```python
from build123d import *

# Parameters (mm, degrees)
SKETCH_W         = 40
SKETCH_H         = 87
PAD_DEPTH        = 5
SKETCH001_R      = 1.35
POCKET_DEPTH     = 10.001
SKETCH009_R      = 1.6
POCKET007_DEPTH  = 10.001
SKETCH010_W      = 5
SKETCH010_H      = 42
POCKET008_DEPTH  = 10.001
CHAMFER_SIZE     = 2
FILLET_R         = 1.5
CHAMFER001_SIZE2 = 1
CHAMFER001_SIZE  = 1
SKETCH011_W      = 22
SKETCH011_H      = 12
POCKET009_DEPTH  = 12
FILLET001_R      = 6
FILLET009_R      = 2
SKETCH012_W      = 27
SKETCH012_H      = 20
POCKET010_DEPTH  = 8
FILLET002_R      = 4
FILLET003_R      = 2
SKETCH013_R      = 10
POCKET011_DEPTH  = 12
SKETCH014_R      = 1.35
POCKET012_DEPTH  = 10.001
SKETCH015_R      = 1.35
POCKET013_DEPTH  = 10.001
SKETCH016_W      = 34
SKETCH016_H      = 34
POCKET014_DEPTH  = 0.5
SKETCH017_R      = 1.35
POCKET015_DEPTH  = 13
FILLET010_R      = 1
FILLET011_R      = 1
SKETCH018_W      = 30
SKETCH018_H      = 2
POCKET016_DEPTH  = 10.001
SKETCH019_R      = 1.35
POCKET017_DEPTH  = 30
SKETCH020_R      = 1.65
POCKET018_DEPTH  = 15
FILLET012_R      = 1
SKETCH021_W      = 0.354353
SKETCH021_H      = 3.81736
PAD001_DEPTH     = 0.2


with BuildPart() as part:
    # Sketch → Pad (new body, symmetric)
    with BuildSketch(Plane.XY):
        Rectangle(SKETCH_W, SKETCH_H)
    extrude(amount=PAD_DEPTH, both=True)

    # Sketch001 (on Face6 of Pad) → Pocket (cut, through all)
    with BuildSketch(Plane.XY.offset(5)):
        with Locations((17, -6.25)):
            Circle(SKETCH001_R)
        with Locations((-11, -6.25)):
            Circle(SKETCH001_R)
        with Locations((-17, -34.25)):
            Circle(SKETCH001_R)
    extrude(amount=-POCKET_DEPTH, mode=Mode.SUBTRACT)

    # Sketch009 (on Face5 of Pocket) → Pocket007 (cut, through all)
    with BuildSketch(Plane.XY.offset(5)):
        with Locations((-16, 3.5)):
            Circle(SKETCH009_R)
        with Locations((-3, 3.5)):
            Circle(SKETCH009_R)
        with Locations((10, 3.5)):
            Circle(SKETCH009_R)
    extrude(amount=-POCKET007_DEPTH, mode=Mode.SUBTRACT)

    # Sketch010 (on Face5 of Pocket007) → Pocket008 (cut, through all)
    with BuildSketch(Plane.XY.offset(5)):
        with Locations((17.5, 22.5)):
            Rectangle(SKETCH010_W, SKETCH010_H)
    extrude(amount=-POCKET008_DEPTH, mode=Mode.SUBTRACT)

    # Chamfer
    chamfer_edges = [part.edges().sort_by_distance(p)[0] for p in [
        (8.4, 3.5, 5),
        (-4.6, 3.5, 5),
        (-17.6, 3.5, 5),
    ]]
    chamfer(chamfer_edges, length=CHAMFER_SIZE)

    # Fillet
    fillet_edges = [part.edges().sort_by_distance(p)[0] for p in [
        (20, 1.5, 0),
        (15, 1.5, 0),
    ]]
    fillet(fillet_edges, radius=FILLET_R)

    # Chamfer001
    chamfer001_edges = [part.edges().sort_by_distance(p)[0] for p in [
        (-20, 43.5, 0),
    ]]
    chamfer001_side = part.faces().sort_by_distance((-2.5, 43.5, 0))[0]
    chamfer(chamfer001_edges, length=CHAMFER001_SIZE, length2=CHAMFER001_SIZE2, reference=chamfer001_side)

    # Sketch011 (on Face1 of Chamfer001) → Pocket009 (cut)
    with BuildSketch(Plane.XY.offset(5)):
        with Locations((3.5, -9.5)):
            Rectangle(SKETCH011_W, SKETCH011_H)
    extrude(amount=-POCKET009_DEPTH, mode=Mode.SUBTRACT)

    # Fillet001
    fillet001_edges = [part.edges().sort_by_distance(p)[0] for p in [
        (-7.5, -3.5, 0),
        (14.5, -15.5, 0),
    ]]
    fillet(fillet001_edges, radius=FILLET001_R)

    # Fillet009
    fillet009_edges = [part.edges().sort_by_distance(p)[0] for p in [
        (14.5, -3.5, 0),
        (-7.5, -15.5, 0),
    ]]
    fillet(fillet009_edges, radius=FILLET009_R)

    # Sketch012 (on Face1 of Fillet001) → Pocket010 (cut)
    with BuildSketch(Plane.XY.offset(5)):
        with Locations((1.5, -28.5)):
            Rectangle(SKETCH012_W, SKETCH012_H)
    extrude(amount=-POCKET010_DEPTH, mode=Mode.SUBTRACT)

    # Fillet002
    fillet002_edges = [part.edges().sort_by_distance(p)[0] for p in [
        (-12, -18.5, 1),
        (-12, -38.5, 1),
        (15, -38.5, 1),
        (15, -18.5, 1),
    ]]
    fillet(fillet002_edges, radius=FILLET002_R)

    # Fillet003
    fillet003_edges = [part.edges().sort_by_distance(p)[0] for p in [
        (-12, -28.5, -3),
    ]]
    fillet(fillet003_edges, radius=FILLET003_R)

    # Sketch013 (on Face4 of Fillet003) → Pocket011 (cut)
    with BuildSketch(Plane.XY.offset(5)):
        with Locations((-3, 29)):
            Circle(SKETCH013_R)
    extrude(amount=-POCKET011_DEPTH, mode=Mode.SUBTRACT)

    # Sketch014 → Pocket012 (cut, through all)
    with BuildSketch(Plane.XY.offset(5)):
        with Locations((-15, 11.5)):
            Circle(SKETCH014_R)
        with Locations((5, 11.5)):
            Circle(SKETCH014_R)
    extrude(amount=-POCKET012_DEPTH, mode=Mode.SUBTRACT)

    # Sketch015 (on Face4 of Pocket012) → Pocket013 (cut, through all)
    with BuildSketch(Plane.XY.offset(5)):
        with Locations((12, -40.5)):
            Circle(SKETCH015_R)
    extrude(amount=-POCKET013_DEPTH, mode=Mode.SUBTRACT)

    # Sketch016 (on Face4 of Pocket013) → Pocket014 (cut)
    with BuildSketch(Plane.XY.offset(5)):
        with Locations((3, -26.5)):
            Rectangle(SKETCH016_W, SKETCH016_H)
    extrude(amount=-POCKET014_DEPTH, mode=Mode.SUBTRACT)

    # Sketch017 (on Face14 of Pocket014) → Pocket015 (cut)
    with BuildSketch(Plane.YZ.offset(20)):
        with Locations((13.5, 0)):
            Circle(SKETCH017_R)
        with Locations((26.5, 0)):
            Circle(SKETCH017_R)
        with Locations((39.5, 0)):
            Circle(SKETCH017_R)
    extrude(amount=-POCKET015_DEPTH, mode=Mode.SUBTRACT)

    # Fillet010
    fillet010_edges = [part.edges().sort_by_distance(p)[0] for p in [
        (20, -43.5, -0.25),
        (-20, -43.5, 0),
        (15, 43.5, 0),
        (-20, 42.5, 0),
        (-19, 43.5, 0),
    ]]
    fillet(fillet010_edges, radius=FILLET010_R)

    # Fillet011
    fillet011_edges = [part.edges().sort_by_distance(p)[0] for p in [
        (20, -9.5, 4.75),
        (14.5, -9.5, 4.75),
        (-7.5, -9.5, 4.75),
        (-14, -9.5, 4.75),
        (-14, -43.5, 4.75),
    ]]
    fillet(fillet011_edges, radius=FILLET011_R)

    # Sketch018 (on Face28 of Fillet011) → Pocket016 (cut, through all)
    with BuildSketch(Plane.XY.offset(5)):
        with Locations((-18, 29)):
            Rectangle(SKETCH018_W, SKETCH018_H)
    extrude(amount=-POCKET016_DEPTH, mode=Mode.SUBTRACT)

    # Sketch019 (on Face49 of Pocket016) → Pocket017 (cut)
    with BuildSketch(Plane(origin=(0, 43.5, 0), x_dir=(-1, 0, 0), z_dir=(0, 1, 0))):
        with Locations((16, 0)):
            Circle(SKETCH019_R)
    extrude(amount=-POCKET017_DEPTH, mode=Mode.SUBTRACT)

    # Sketch020 (on Face50 of Pocket017) → Pocket018 (cut)
    with BuildSketch(Plane(origin=(0, 43.5, 0), x_dir=(-1, 0, 0), z_dir=(0, 1, 0))):
        with Locations((16, 0)):
            Circle(SKETCH020_R)
    extrude(amount=-POCKET018_DEPTH, mode=Mode.SUBTRACT)

    # Fillet012
    fillet012_edges = [part.edges().sort_by_distance(p)[0] for p in [
        (-12.949874, 28, 0),
        (-12.949874, 30, 0),
        (-20, 28, 0),
        (-20, 30, 0),
    ]]
    fillet(fillet012_edges, radius=FILLET012_R)

    # Sketch021 (on Face43 of Fillet012) → Pad001 (join)
    with BuildSketch(Plane(origin=(0, 0, -5), x_dir=(1, 0, 0), z_dir=(0, 0, -1))):
        with Locations((-18.602508, -29.247387)):
            Rectangle(SKETCH021_W, SKETCH021_H)
    extrude(amount=-PAD001_DEPTH)


solid = part.part
```
The model under review builds one solid part; all positions refer to its coordinate system, in mm. A direction names the side the tool comes from. Give positions to 0.01 mm unless a question says otherwise; leave off trailing zeros. Write each loop counter-clockwise with the first axis right and the second up, starting at its lowest first coordinate (ties: lowest second). Pieces come first, ordered by that corner, then holes. Notation, with made-up numbers: M -32.5,-5 L -20.5,-5 A25 ccw -20.5,26 Z; hole C 18,82 d5. An arc over 180 degrees is marked long. Write item = value, one per line. Start each with the question number.
Q1. Mouldability with a two-part tool opening along Y and no side actions: class faces 5 (the face through (0, -43.5, 0)), 6 (the face through (-4.18, 4.58, -0.94)), 7 (the face through (-17.574, 36.844, 0.496)) as released by +Y, released by -Y, zero draft, split by the parting line, or undercut.
Q2. We need section A-A (y = -29.5). State the section outline as (x, z) points.
Q3. Machinability: for faces 1 (the face through (14.43, -28.58, -2.4)), 2 (the face through (14.5, -8, 0)), 3 (the face through (2, -18, 4.5)), 4 (the face through (11.06, 38.15, 0.06)), which of the approach directions +Z, -Z, +X, -X, +Y, -Y give a long, thin tool a straight path to every point of the face, cutting with its end or side? Answer none if there is none.
Q4. For line 1 (Z direction, x = -16, y = 18); line 2 (Y direction, x = 2, z = 1.75); line 3 (Y direction, x = -3.5, z = -3.25), list the stretches that pass through material, from the lowest coordinate up.
Q5. Clearance check with flat-ended pins moving along their axes: pin 1 (12 mm diameter, centred on x = -3, y = 29, fed in from -Z); pin 2 (1.5 mm diameter, centred on y = 19.5, z = -2, fed in from +X); pin 3 (3.5 mm diameter, centred on x = 10, y = 3.5, fed in from -Z). State where each tip first meets the part, or that it passes through.
Result set:
q1.face_5 = released by -Y
q1.face_6 = undercut
q1.face_7 = zero draft
q2.outline = M -20,-5 L 20,-5 L 20,4.5 L 15,4.5 L 15,-1 A2 cw 13,-3 L -10,-3 A2 cw -12,-1 L -12,4.5 L -14,4.5 L -14,5 L -20,5 Z
q3.face_1 = +Z
q3.face_2 = +Z, -Z
q3.face_3 = +Z, +X, -Y
q3.face_4 = +X
q4.line_1 = -5 to -1.35, 1.35 to 5
q4.line_2 = -43.5 to -38.5, -18.5 to -15.5, -3.5 to 20.34, 37.66 to 43.5
q4.line_3 = -43.5 to -15.5, -3.84 to 1.98, 5.02 to 19.01, 38.99 to 43.5
q5.pin_1 = through
q5.pin_2 = 15
q5.pin_3 = -5
